```python
from build123d import *

# Parameters (mm, degrees)
F0_W     = 120
F0_H     = 30
F0_R     = 5
F1_DEPTH = 6
F2_W     = 40
F2_H     = 30
F3_DEPTH = 35
F5_DEPTH = 122


with BuildPart() as f1:
    # F0 (on Top) → F1 (new body)
    with BuildSketch(Plane.XY):
        Rectangle(F0_W, F0_H)
        Circle(F0_R, mode=Mode.SUBTRACT)
    extrude(amount=F1_DEPTH)

    # F2 (on face) → F3 (join)
    with BuildSketch(Plane.XY.offset(6)):
        with Locations((-40, 0)):
            Rectangle(F2_W, F2_H)
        with Locations((40, 0)):
            Rectangle(F2_W, F2_H)
    extrude(amount=F3_DEPTH)

    # F4 (on face) → F5 (cut)
    with BuildSketch(Plane.YZ.offset(60)):
        with BuildLine():
            Line((0, 41), (-15, 41))
            Line((-15, 41), (-15, 26))
            ThreePointArc((-15, 26), (-10.606602, 36.606602), (0, 41))
        make_face()
        with BuildLine():
            Line((15, 41), (0, 41))
            ThreePointArc((0, 41), (10.606602, 36.606602), (15, 26))
            Line((15, 26), (15, 41))
        make_face()
        with BuildLine():
            ThreePointArc((4, 26), (2.828427, 28.828427), (0, 30))
            ThreePointArc((0, 30), (-2.828427, 23.171573), (4, 26))
        make_face()
    extrude(amount=-F5_DEPTH, mode=Mode.SUBTRACT)


solid = f1.part
```
CAD build for the part. Positions are in the model's coordinates, mm. A direction names the side the tool comes from. Give positions to 0.01 mm unless a question says otherwise; leave off trailing zeros. Order: outer loops, then holes, each group sorted by start corner. A loop starts at its lowest first (then second) coordinate and runs counter-clockwise, first axis right, second up. Notation, with made-up numbers: M 32,-14 L 81,-14 A20 cw 81,13 Z; hole C 59.25,54.5 d3. An arc over 180 degrees is marked long. Put each result on its own line as item: value. Start each with the question number.
(1) Saw through at B-B, the plane z = 14. Write the cut outline in (x, y), then the cut area to 3 significant figures.
(2) Saw through at C-C, the plane y = -2.5. Write the cut outline in (x, z), then the cut area to 3 significant figures.
(3) Saw through at A-A, the plane x = -45.5. Write the cut outline in (y, z).
(4) Mould opens along Y. For faces 1 (the cylindrical face through (-1.08, -4.88, 2.96)), 2 (the flat face through (-20, 0, 19)), 3 (the flat face through (-1, -15, 4)), 4 (the flat face through (-1, 15, 4)) say: +Y half, -Y half, draft (parallel to the pull), parting line (faces both ways), or undercut.
(5) Flat gauge pin, fed straight in: pin 1 Ø5 at (y, z) = (0, 26) entering from -X. Where does the tip first touch, or does it go through?
(6) Saw through at D-D, the plane x = 0. Write the cut outline in (y, z), then the cut area to 3 significant figures.
(7) Drill centre lines: line 1 along Y through (x, z) = (-41, 26); line 2 along X through (y, z) = (11.5, 14); line 3 along Z through (x, y) = (-28, 0). Where is each one in solid material? Low to high.
(8) Which spindle directions (+Z, -Z, +X, -X, +Y, -Y) get a long thin tool onto all of the face, cutting with end or side? Do faces 5 (the flat face through (-5, 4, 6)), 6 (the flat face through (60, 0, 20)). Say none if no direction does.
Check result:
1. outline: M -60,-15 L -20,-15 L -20,15 L -60,15 Z; M 20,-15 L 60,-15 L 60,15 L 20,15 Z
1. area: 2,400 mm2
2. outline: M -60,0 L -4.33,0 L -4.33,6 L -20,6 L -20,22.88 L -60,22.88 Z; M -60,29.12 L -20,29.12 L -20,40.79 L -60,40.79 Z; M 4.33,0 L 60,0 L 60,22.88 L 20,22.88 L 20,6 L 4.33,6 Z; M 20,29.12 L 60,29.12 L 60,40.79 L 20,40.79 Z
2. area: 2,950 mm2
3. outline: M -15,0 L 15,0 L 15,26 A15 ccw 0,41 A15 ccw -15,26 Z; hole C 0,26 d8
4. face 1: undercut
4. face 2: draft
4. face 3: -Y half
4. face 4: +Y half
5. pin 1: passes through
6. outline: M -15,0 L -5,0 L -5,6 L -15,6 Z; M 5,0 L 15,0 L 15,6 L 5,6 Z
6. area: 120 mm2
7. line 1: y = -15 to -4, 4 to 15
7. line 2: x = -60 to -20, 20 to 60
7. line 3: z = 0 to 22, 30 to 41
8. face 5: +Z, +Y, -Y
8. face 6: +Z, -Z, +X, +Y, -Y
